Source: CAD feature listing. Evaluate the final solid. Frame: model axes, mm. A direction names the side the tool comes from. Round coordinates to 2 decimals unless told otherwise and drop trailing zeros. Loops run counter-clockwise (first coordinate to the right, second up) from the corner with the lowest first, then second, coordinate; pieces in that order, holes last. Notation, with made-up numbers: M 21,81.5 L 70,81.5 A20 cw 70,104.5 Z; hole C 56.25,55.25 d11. An arc over 180 degrees is marked long. Answer as a JSON object with one key per item and string values.
from build123d import *

# Parameters (mm, degrees)
F0_W      = 158.75
F0_H      = 70.485
F1_DEPTH  = 104.775
F2_T      = -3.175
F3_W      = 152.4
F3_H      = 64.135
F4_DEPTH  = 3.175
F5_W      = 152.4
F5_H      = 3.175
F6_DEPTH  = 104.775
F7_W      = 107.95
F7_H      = 3.175
F8_DEPTH  = 104.775
F9_W      = 158.75
F9_H      = 70.485
F9_W_2    = 107.95
F9_H_2    = 51.435
F10_DEPTH = 3.175
F11_R     = 6.35
F12_W     = 101.6
F12_H     = 76.2
F13_DEPTH = 3.175
F14_R     = 12.7


with BuildPart() as f1:
    # F0 (on Front) → F1 (new body)
    with BuildSketch(Plane.XZ):
        Rectangle(F0_W, F0_H)
    extrude(amount=-F1_DEPTH)

    # F2
    f2_openings = [f1.faces().sort_by_distance(p)[0] for p in [
        (0, 0, 0),
    ]]
    offset(amount=F2_T, openings=f2_openings)

    # F3 (on face) → F4 (cut, through all)
    with BuildSketch(Plane.XZ.offset(-101.6)):
        Rectangle(F3_W, F3_H)
    extrude(amount=-F4_DEPTH, mode=Mode.SUBTRACT)

    # F5 (on face) → F6 (join)
    with BuildSketch(Plane.XZ):
        Rectangle(F5_W, F5_H)
    extrude(amount=-F6_DEPTH)

    # F7 (on face) → F8 (cut, through all)
    with BuildSketch(Plane.XZ):
        Rectangle(F7_W, F7_H)
    extrude(amount=-F8_DEPTH, mode=Mode.SUBTRACT)

    # F9 (on face) → F10 (join)
    with BuildSketch(Plane(origin=(0, 104.775, 0), x_dir=(-1, 0, 0), z_dir=(0, 1, 0))):
        Rectangle(F9_W, F9_H)
        Rectangle(F9_W_2, F9_H_2, mode=Mode.SUBTRACT)
    extrude(amount=F10_DEPTH)

    # F11
    f11_edges = [f1.edges().sort_by_distance(p)[0] for p in [
        (53.975, 106.3625, 25.7175),
        (-53.975, 106.3625, 25.7175),
        (-53.975, 106.3625, -25.7175),
        (53.975, 106.3625, -25.7175),
    ]]
    fillet(f11_edges, radius=F11_R)

    # F12 (on face) → F13 (cut, through all)
    with BuildSketch(Plane(origin=(0, 0, -35.2425), x_dir=(1, 0, 0), z_dir=(0, 0, -1))):
        with Locations((0, -38.1)):
            Rectangle(F12_W, F12_H)
    extrude(amount=-F13_DEPTH, mode=Mode.SUBTRACT)

    # F14
    f14_edges = [f1.edges().sort_by_distance(p)[0] for p in [
        (-50.8, 76.2, -33.655),
        (50.8, 76.2, -33.655),
    ]]
    fillet(f14_edges, radius=F14_R)


solid = f1.part
Item 1: Section C-C on z = 6. Return the cut outline in (x, y) (3 decimals), then the cut area to 3 significant figures.
Answer sheet:
{"outline": "M -79.375,0 L -76.2,0 L -76.2,104.775 L -53.975,104.775 L -53.975,107.95 L -79.375,107.95 Z; M 53.975,104.775 L 76.2,104.775 L 76.2,0 L 79.375,0 L 79.375,107.95 L 53.975,107.95 Z", "area": "827 mm²"}
Item 2: Section B-B on y = 83.5. Return the cut outline in (x, z) (1 decimal).
Answer sheet:
{"outline": "M -79.4,-35.2 L 79.4,-35.2 L 79.4,35.2 L -79.4,35.2 Z; hole M -76.2,-32.1 L 76.2,-32.1 L 76.2,-1.6 L 54,-1.6 L 54,1.6 L 76.2,1.6 L 76.2,32.1 L -76.2,32.1 L -76.2,1.6 L -54,1.6 L -54,-1.6 L -76.2,-1.6 Z"}
Item 3: Contact query for flat-ended pins moving along their axis: pin 1 Ø2 at (x, z) = (19.5, -27.5) entering from -Y (3 decimals); pin 2 Ø1.6 at (x, z) = (-9, -33.5) entering from -Y. Output: stop coordinate, or through.
Answer sheet:
{"pin 1": "stops at y = 104.775", "pin 2": "stops at y = 76.2"}
Item 4: Pull-direction query (X, two-part tool) for faces 1 (the flat face through (-79.375, 53, 0)), 2 (the cylindrical face through (52.065, 106.385, 23.907)), 3 (the flat face through (19, 107.95, -31)); classes: pulls with the +X half, pulls with the -X half, needs draft (parallel to the pull), parting line crosses it, or undercut.
Answer sheet:
{"face 1": "pulls with the -X half", "face 2": "undercut", "face 3": "needs draft"}
Item 5: Section D-D on y = 14. Return the cut outline in (x, z) (1 decimal), then the cut area to 3 significant figures.
Answer sheet:
{"outline": "M -79.4,-35.2 L -50.8,-35.2 L -50.8,-32.1 L -76.2,-32.1 L -76.2,-1.6 L -54,-1.6 L -54,1.6 L -76.2,1.6 L -76.2,32.1 L 76.2,32.1 L 76.2,1.6 L 54,1.6 L 54,-1.6 L 76.2,-1.6 L 76.2,-32.1 L 50.8,-32.1 L 50.8,-35.2 L 79.4,-35.2 L 79.4,35.2 L -79.4,35.2 Z", "area": "1,230 mm²"}
Item 6: Line query: probe 1 along Z at (x, y) = (-62, 88); probe 2 along X at (y, z) = (101, 15) (3 decimals); probe 3 along Z at (x, y) = (8, 77.5). Output: solid intervals per line, ascending. Write a range as from..to.
Answer sheet:
{"probe 1": "z = -35.24..-32.07, -1.59..1.59, 32.07..35.24", "probe 2": "x = -79.375..-76.2, 76.2..79.375", "probe 3": "z = -35.24..-32.07, 32.07..35.24"}
Item 7: Access query for faces 4 (the flat face through (53.975, 66, 0)), 5 (the cylindrical face through (-47.18, 72.38, -33.63)), 6 (the flat face through (-65, 52, 1.588)). Directions: +Z, -Z, +X, -X, +Y, -Y. A direction counts if a zero-diameter tool reaches every point of the face in a straight line with its end or side. Return the directions, or none.
Answer sheet:
{"face 4": "+Y, -Y", "face 5": "-Z, -Y", "face 6": "-Y"}
